Can you work these out from the drawing? Everything is in mm from the part's minimum corner. Give positions to 0.01 mm unless a question says otherwise; leave off trailing zeros. Order: outer loops, then holes, each group sorted by start corner. A loop starts at its lowest first (then second) coordinate and runs counter-clockwise, first axis right, second up. Notation, with made-up numbers: (26.5, 70.5) - (33.5, 70.5) arc R25 ccw to (33.5, 82.5) - close; hole circle Ø4 at (59, 19.25). An arc over 180 degrees is marked (long way). Write each question's results on one line, items separated by ' | '. Start each with the question number.
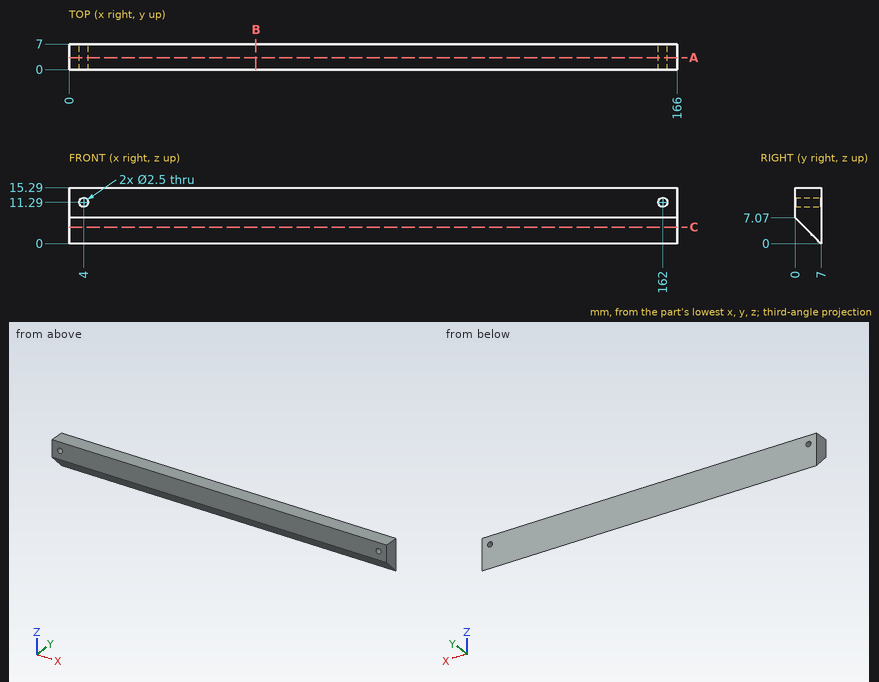
Q1. If I drill on probe 1 along X at (y, z) = (3.5, 11.29); probe 2 along Z at (x, y) = (4, 4); probe 3 along Z at (x, y) = (4, 5), over which ranges is the centre line in solid material (lowest first)? Write a range as from..to.
Q2. If we section it at B-B (x = 51): Please give me the cut outline in (y, z).
Q3. Will these pins go through, and if not, where does the flat tip stop? P1, Ø3, axis at x = 162, z = 11.29, coming from the +Y side; P2, Ø1, axis at x = 35.5, y = 4.5, coming from the -Z side.
Q4. If we section it at A-A (y = 3.25): Please give me the cut outline in (x, z).
Q5. If we section it at C-C (z = 4.5): Please give me the cut outline in (x, y), plus the area to 3 significant figures.
Findings below:
1) probe 1: x = 0..2.75, 5.25..160.75, 163.25..166 | probe 2: z = 3.03..10.04, 12.54..15.29 | probe 3: z = 2.02..10.04, 12.54..15.29
2) outline: (0, 7.07) - (7, 0) - (7, 15.29) - (0, 15.29) - close
3) P1: stops at y = 7 | P2: stops at z = 2.02
4) outline: (0, 3.79) - (166, 3.79) - (166, 15.29) - (0, 15.29) - close; hole circle Ø2.5 at (4, 11.29); hole circle Ø2.5 at (162, 11.29)
5) outline: (0, 2.54) - (166, 2.54) - (166, 7) - (0, 7) - close | area: 740 mm2
